Autodesk Fusion 360 part; units mm, degrees
sketch "草图1" plane through (0, 0, 0) normal (0, 1, 0) x (1, 0, 0)
  line L0 (4, 0) -> (12.5, 0)
  line L1 (16.5, -4) -> (16.5, -40)
  line L2 (12.5, -44) -> (4, -44)
  line L3 (0, -40) -> (0, -4)
  arc A0 (0, -40) -> (4, -44) centre (4, -40) ccw
  arc A1 (12.5, -44) -> (16.5, -40) centre (12.5, -40) ccw
  arc A2 (16.5, -4) -> (12.5, 0) centre (12.5, -4) ccw
  arc A3 (4, 0) -> (0, -4) centre (4, -4) ccw
  point P0 (16.5, 0)
  point P1 (0, -44)
  dimension "d3" = 4
  dimension "d4" = 4
  dimension "d5" = 4
  dimension "d6" = 4
  dimension "d8" = 44
  dimension "d9" = 16.5
extrude "拉伸1" add sketch "草图1" along normal blind 12 makes body 1
fillet "圆角1" radius 2 8 edges at (16.5, 12, 22) (15.3284, 12, 1.1716) (8.25, 12, 0) (1.1716, 12, 1.1716) (0, 12, 22) (1.1716, 12, 42.8284) (8.25, 12, 44) (15.3284, 12, 42.8284) on bodies 1
fillet "圆角2" radius 2 8 edges at (1.1716, 0, 42.8284) (0, 0, 22) (1.1716, 0, 1.1716) (8.25, 0, 0) (15.3284, 0, 1.1716) (16.5, 0, 22) (15.3284, 0, 42.8284) (8.25, 0, 44) on bodies 1
sketch "草图2" plane through (0, 0, 0) normal (0, -1, 0) x (1, 0, 0)
  arc A0 (4, 42) -> (2, 40) centre (4, 40) ccw
  line L0 (2, 40) -> (2, 4)
  arc A1 (2, 4) -> (4, 2) centre (4, 4) ccw
  line L1 (4, 2) -> (12.5, 2)
  arc A2 (12.5, 2) -> (14.5, 4) centre (12.5, 4) ccw
  line L2 (14.5, 4) -> (14.5, 40)
  arc A3 (14.5, 40) -> (12.5, 42) centre (12.5, 40) ccw
  line L3 (12.5, 42) -> (4, 42)
  circle A4 centre (8.25, 22) radius 5
  dimension "d16" = 10
  dimension "d17" = 6.25
  dimension "d18" = 20
extrude "拉伸2" cut sketch "草图2" against normal blind 2 contours A4 bodies 1
chamfer "倒角1" distance 1 angle 45 1 faces at (13.2438, 1.3333, 21.7508) on bodies 1
sketch "草图3" plane through (0, 2, 0) normal (0, -1, 0) x (1, 0, 0)
  circle A0 centre (8.25, 22) radius 4
  circle A1 centre (8.25, 22) radius 4
  circle A2 centre (8.25, 22) radius 3
  dimension "d22" = 6
extrude "拉伸3" add sketch "草图3" along normal blind 2 bodies 1
extrude "拉伸4" add 1 faces at (7.75, 2, 22.9957) along direction (0, -1, 0) blind 6.5 on bodies 1 bodies 1
sketch "草图4" plane through (0, 0, 0) normal (0, 0, -1) x (1, 0, 0)
  line L0 (12.5, -2) -> (4, -2)
  line L1 (4, -2) -> (4, -10)
  line L2 (4, -10) -> (12.5, -10)
  line L3 (12.5, -10) -> (12.5, -2)
  circle A0 centre (8.25, -6) radius 1.5
  dimension "d27" = 3
  dimension "d29" = 4.25
  dimension "d30" = 4
extrude "拉伸5" add sketch "草图4" along normal blind 2 contours A0 bodies 1
sketch "草图5" plane through (0, 0, 44) normal (0, 0, 1) x (-1, 0, 0)
  line L0 (-4, -2) -> (-12.5, -2)
  line L1 (-12.5, -2) -> (-12.5, -10)
  line L2 (-12.5, -10) -> (-4, -10)
  line L3 (-4, -10) -> (-4, -2)
  circle A0 centre (-8.25, -6) radius 1.5
  dimension "d33" = 3
  dimension "d34" = 4
  dimension "d35" = 4.25
extrude "拉伸6" add sketch "草图5" along normal blind 2 contours A0 bodies 1
copy_body "实体->零部件1" bodies 1 removing the originals makes body 2 in component "Component'"
component "Component'" placed x (1, 0, 0) y (0, 1, 0) z (0, 0, 1) at (0, 0, 0)
The listing builds one solid part. Answer for the finished solid, in the listing's coordinates (mm). A direction names the side the tool comes from. Give positions to 0.01 mm unless a question says otherwise; leave off trailing zeros. Order: outer loops, then holes, each group sorted by start corner. A loop starts at its lowest first (then second) coordinate and runs counter-clockwise, first axis right, second up. Notation, with made-up numbers: (50.5, 41.5) - (76.5, 41.5) arc R25 ccw to (76.5, 79.5) - close; hole circle Ø4 at (-39, 60.5). An arc over 180 degrees is marked (long way). Answer in a Markdown table with one row per item. Add a question column.
Q1. The part is cut by section D-D (y = 6). Determine the outline of the cut face in (x, z).
Q2. The part is cut by section B-B (z = 9). Determine the outline of the cut face in (x, y).
Q3. Given P1, Ø5, axis at x = 3.5, z = 38, coming from the -Y side; P2, Ø1, axis at y = 0.5, z = 35, coming from the -X side, each flat-ended and moving along its own axis, determine where each tip first touches the part or whether it passes through.
Q4. The part is cut by section A-A (y = 8.25). Determine the outline of the cut face in (x, z).
Q5. Find the intervals of material crossed by line 1 along Z through (x, y) = (7, 10); line 2 along Z through (x, y) = (8.25, 1); line 3 along Y through (x, z) = (13, 33), in increasing order. Write a range as [from, to].
Q6. Which of the six approach directions +Z, -Z, +X, -X, +Y, -Y give full straight-line access (tool end or side, diameter ignored) to faces 1 (the flat face through (8, 4, 0)), 2 (the flat face through (8, 12, 22)), 3 (the cylindrical face through (11.02, -2.22, 23.15))?
Determined:
| question | item | result |
|---|---|---|
| 1 | outline | (0, 4) arc R4 ccw to (4, 0) - (6.75, 0) - (6.75, -2) - (9.75, -2) - (9.75, 0) - (12.5, 0) arc R4 ccw to (16.5, 4) - (16.5, 40) arc R4 ccw to (12.5, 44) - (9.75, 44) - (9.75, 46) - (6.75, 46) - (6.75, 44) - (4, 44) arc R4 ccw to (0, 40) - close |
| 2 | outline | (0, 2) arc R2 ccw to (2, 0) - (14.5, 0) arc R2 ccw to (16.5, 2) - (16.5, 10) arc R2 ccw to (14.5, 12) - (2, 12) arc R2 ccw to (0, 10) - close |
| 3 | P1 | stops at y = 0 |
| 3 | P2 | stops at x = 0.27 |
| 4 | outline | (0, 4) arc R4 ccw to (4, 0) - (12.5, 0) arc R4 ccw to (16.5, 4) - (16.5, 40) arc R4 ccw to (12.5, 44) - (4, 44) arc R4 ccw to (0, 40) - close |
| 5 | line 1 | z = [0, 44] |
| 5 | line 2 | z = [0.27, 17], [18, 26], [27, 43.73] |
| 5 | line 3 | y = [0, 12] |
| 6 | face 1 | -Z |
| 6 | face 2 | +Z, -Z, +X, -X, +Y |
| 6 | face 3 | -Y |
